Work out the finished part from the listing and answer in its coordinate system (mm). Coordinates: 2 decimals unless noted, no trailing zeros. Order: outer loops, then holes, each group sorted by start corner. A loop starts at its lowest first (then second) coordinate and runs counter-clockwise, first axis right, second up. Notation, with made-up numbers: M 19.25,-25 L 27.25,-25 A9 ccw 27.25,-18 Z; hole C -31.75,15.5 d9. An arc over 180 degrees is marked long. Use a Markdown table: item, result.
from build123d import *

# Parameters (mm, degrees)
F1_DEPTH = 103.1875
F2_R     = 3.175
F3_DEPTH = 103.1885


with BuildPart() as f1:
    # F0 (on Right) → F1 (new body)
    with BuildSketch(Plane.YZ):
        Polygon((3.666174, 6.35), (-3.666174, 6.35), (-7.332348, 0), (-3.666174, -6.35), (3.666174, -6.35), (7.332348, 0), align=None)
    extrude(amount=F1_DEPTH)

    # F2 (on face) → F3 (cut, through all)
    with BuildSketch(Plane.YZ.offset(103.1875)):
        Circle(F2_R)
    extrude(amount=-F3_DEPTH, mode=Mode.SUBTRACT)


solid = f1.part
(1) A cutting plane is placed at D-D (z = -4.25). Determine the outline of the cut face in (x, y), then the cut area to 3 significant figures.
Conclusion:
| item | result |
|---|---|
| outline | M 0,-4.88 L 103.19,-4.88 L 103.19,4.88 L 0,4.88 Z |
| area | 1,010 mm2 |
(2) Given P1, Ø6, axis at x = 33, z = -3.5, coming from the -Y side, flat-ended and moving along its own axis, determine where the tip first touches the part or whether it passes through.
Conclusion:
| item | result |
|---|---|
| P1 | y = -7.04 |
(3) Straight lines are drawn through the part: L1, parallel to Z at x = 36, y = 0 (3 decimals); L2, parallel to Y at x = 5.5, z = 1 (3 decimals); L3, parallel to Z at x = 8, y = 0.5. For each, find the intervals that lie inside material, in ascending order.
Conclusion:
| item | result |
|---|---|
| L1 | -6.35 to -3.175, 3.175 to 6.35 |
| L2 | -6.755 to -3.013, 3.013 to 6.755 |
| L3 | -6.35 to -3.14, 3.14 to 6.35 |
(4) A cutting plane is placed at C-C (z = 1.25). Determine the outline of the cut face in (x, y).
Conclusion:
| item | result |
|---|---|
| outline | M 0,-6.61 L 103.19,-6.61 L 103.19,-2.92 L 0,-2.92 Z; M 0,2.92 L 103.19,2.92 L 103.19,6.61 L 0,6.61 Z |
(5) Determine the mould class of faces 1 (the flat face through (103.188, 2, 3)), 2 (the flat face through (50.871, 5.474, -3.219)), 3 (the cylindrical face through (52.32, -0.69, -3.1)) for opening direction Z: pulls with the +Z half, pulls with the -Z half, needs draft (parallel to the pull), parting line crosses it, or undercut.
Conclusion:
| item | result |
|---|---|
| face 1 | needs draft |
| face 2 | pulls with the -Z half |
| face 3 | undercut |
(6) A cutting plane is placed at A-A (x = 31.5). Determine the outline of the cut face in (y, z) (3 decimals), then the cut area to 3 significant figures.
Conclusion:
| item | result |
|---|---|
| outline | M -7.332,0 L -3.666,-6.35 L 3.666,-6.35 L 7.332,0 L 3.666,6.35 L -3.666,6.35 Z; hole C 0,0 d6.35 |
| area | 108 mm2 |
